```python
from build123d import *
from build123d.topology import SkipClean

# Parameters (mm, degrees)
EXTRUDE_1_DEPTH          = 2.5
EXTRUDE_START            = -3
SKETCH_1_4_R             = 4
EXTRUDE_2_DEPTH          = 3
CUT_EXTRUDE_1_DEPTH      = 44.965895874
CUT_EXTRUDE_1_DEPTH_BACK = 44.965895874
SKETCH_1_3_R             = 2
SKETCH_2_R               = 3
CUT_EXTRUDE_2_DEPTH      = 1.5
CUT_EXTRUDE_START        = -2.5
SKETCH_2_3_R             = 3
CUT_EXTRUDE_3_DEPTH      = 1.5
SKETCH_3_W               = 7.983418506
SKETCH_3_H               = 52.149860593
CUT_EXTRUDE_4_DEPTH      = 45.988887517


with BuildPart() as part:
    # 草图1 → 凸台-拉伸1 (new body)
    with BuildSketch(Plane(origin=(0, 0, 0), x_dir=(0, 0, -1), z_dir=(1, 0, 0))):
        with BuildLine():
            Line((17.391993216, -17.88000424), (7.391993216, -1.88000424))
            ThreePointArc((7.391993216, -1.88000424), (2.897269948, -0.155005015), (0, -4))
            Line((0, -4), (0, -36))
            ThreePointArc((0, -36), (2.897269948, -39.844994985), (7.391993216, -38.11999576))
            Line((7.391993216, -38.11999576), (17.391993216, -22.11999576))
            ThreePointArc((17.391993216, -22.11999576), (18, -20), (17.391993216, -17.88000424))
        make_face()
    extrude(amount=EXTRUDE_1_DEPTH)

    # 草图1<4> → 凸台-拉伸2 (add)
    with SkipClean():  # the faces are left unmerged after this step: merging them gives an invalid solid
        with BuildSketch(Plane(origin=(0, 0, 0), x_dir=(0, 0, -1), z_dir=(1, 0, 0)).offset(EXTRUDE_START)):
            with Locations(Location((4, -4, 0), (0, 0, 180))):
                Circle(SKETCH_1_4_R)
        extrude(amount=EXTRUDE_2_DEPTH)

    # 草图1<3> → 切除-拉伸1 (cut, two sides: drawn at the far end of the back side and taken through both)
    with SkipClean():  # the faces are left unmerged after this step: merging them gives an invalid solid
        with BuildSketch(Plane(origin=(0, 0, 0), x_dir=(0, 0, -1), z_dir=(1, 0, 0)).offset(-CUT_EXTRUDE_1_DEPTH_BACK)):
            with Locations((4, -4)):
                Circle(SKETCH_1_3_R)
            with Locations((14, -20)):
                Circle(SKETCH_1_3_R)
            with Locations((4, -36)):
                Circle(SKETCH_1_3_R)
        extrude(amount=CUT_EXTRUDE_1_DEPTH + CUT_EXTRUDE_1_DEPTH_BACK, mode=Mode.SUBTRACT)

    # 草图2 → 切除-拉伸2 (cut)
    with SkipClean():  # the faces are left unmerged after this step: merging them gives an invalid solid
        with BuildSketch(Plane(origin=(2.5, 0, 0), x_dir=(0, 0, -1), z_dir=(1, 0, 0))):
            with Locations((4, -4)):
                Circle(SKETCH_2_R)
            with Locations((14, -20)):
                Circle(SKETCH_2_R)
        extrude(amount=-CUT_EXTRUDE_2_DEPTH, mode=Mode.SUBTRACT)

    # 草图2<3> → 切除-拉伸3 (cut)
    with SkipClean():  # the faces are left unmerged after this step: merging them gives an invalid solid
        with BuildSketch(Plane(origin=(2.5, 0, 0), x_dir=(0, 0, -1), z_dir=(1, 0, 0)).offset(CUT_EXTRUDE_START)):
            with Locations((4, -36)):
                Circle(SKETCH_2_3_R)
        extrude(amount=CUT_EXTRUDE_3_DEPTH, mode=Mode.SUBTRACT)


with BuildPart() as body_2:
    # 镜向2: mirrored copy
    add(part.part.mirror(Plane(origin=(3.5, 0, 0), x_dir=(0, 0, 1), z_dir=(1, 0, 0))))


with BuildPart() as part_1:
    add(part.part)

    # 草图3 → 切除-拉伸4 (cut, through all)
    with BuildSketch(Plane.XY):
        with Locations((-0.565425098, -20.529857361)):
            Rectangle(SKETCH_3_W, SKETCH_3_H)
    extrude(amount=-CUT_EXTRUDE_4_DEPTH, mode=Mode.SUBTRACT)


solid = body_2.part
```
Here's how the part is built. I have some questions about the finished solid (model axes, mm). A direction names the side the tool comes from. Give positions to 0.01 mm unless a question says otherwise; leave off trailing zeros. Loops run counter-clockwise (first coordinate to the right, second up) from the corner with the lowest first, then second, coordinate; pieces in that order, holes last. Notation, with made-up numbers: M 19.5,-37.75 L 75.5,-37.75 A30 ccw 75.5,-14.75 Z; hole C 65,40.25 d2. An arc over 180 degrees is marked long. Put each result on its own line as item: value. Start each with the question number.
(1) For faces 1 (the flat face through (6, -5, -6)), 2 (the cylindrical face through (6.26, -33.97, -1.79)), 3 (the flat face through (5.768, -30.232, -12.322)), which set-ups out of +Z, -Z, +X, -X, +Y, -Y let a thin tool reach every point of the face, with its end or its side?
(2) Will these pins go through, and if not, where does the flat tip stop? pin 1 Ø5 at (y, z) = (-20, -14) entering from -X; pin 2 Ø8 at (y, z) = (-10.5, -13) entering from +X.
(3) I need wall thicknesses on line 1 along Y through (x, z) = (4.9, -4); line 2 along Y through (x, z) = (6.3, -5.25); line 3 along Z through (x, y) = (6.3, -20). Which ranges of each line are inside material? Lowest first, please. Write a range as [from, to].
(4) I want a section at B-B on y = -20. Please give me the cut outline in (x, z), then the cut area to 3 significant figures.
(5) If we mould it in two halves opening along Y, with no side actions, what happens to faces 4 (the cylindrical face through (5.2, -21.8, -11.6)), 5 (the cylindrical face through (6, -20, -18)), 6 (the flat face through (4.5, -20, -7)), 7 (the flat face through (5.77, -9.99, -12.46))? For each: +Y half, -Y half, draft (parallel to the pull), parting line (faces both ways), or undercut.
(6) I want a section at C-C on x = 6.45. Please give me the cut outline in (y, z).
(7) I want a section at A-A on z = -4. Please give me the cut outline in (x, y).
(8) I want a section at D-D on z = -14. Please give me the cut outline in (x, y), then the cut area to 3 significant figures.
Answer block:
1. face 1: -X
1. face 2: +X
1. face 3: -Z, +X, -X, -Y
2. pin 1: x = 6
2. pin 2: x = 7
3. line 1: [-40, -38], [-34, -7], [-1, 0]
3. line 2: [-39.8, -38.73], [-33.27, -5.56], [-2.44, -0.2]
3. line 3: [-18, -16], [-12, 0]
4. outline: M 4.5,-18 L 7,-18 L 7,-16 L 6,-16 L 6,-17 L 4.5,-17 Z; M 4.5,-11 L 6,-11 L 6,-12 L 7,-12 L 7,0 L 4.5,0 Z
4. area: 32.0 mm^2
5. face 4: undercut
5. face 5: parting line
5. face 6: draft
5. face 7: +Y half
6. outline: M -38.12,-7.39 L -22.12,-17.39 A4 ccw -17.88,-17.39 L -1.88,-7.39 A4 ccw -4,0 L -36,0 A4 ccw Z; hole C -36,-4 d6; hole C -20,-14 d4; hole C -4,-4 d4
7. outline: M 4.5,-40 L 7,-40 L 7,-39 L 5.5,-39 L 5.5,-38 L 4.5,-38 Z; M 4.5,-34 L 5.5,-34 L 5.5,-33 L 7,-33 L 7,-8 L 10,-8 L 10,-6 L 6,-6 L 6,-7 L 4.5,-7 Z; M 4.5,-1 L 6,-1 L 6,-2 L 10,-2 L 10,0 L 4.5,0 Z
8. outline: M 4.5,-27.55 L 7,-27.55 L 7,-22 L 6,-22 L 6,-23 L 4.5,-23 Z; M 4.5,-17 L 6,-17 L 6,-18 L 7,-18 L 7,-12.45 L 4.5,-12.45 Z
8. area: 24.7 mm^2
